The model under review builds one solid part; all positions refer to its coordinate system, in mm. A direction names the side the tool comes from. Round coordinates to 2 decimals unless told otherwise and drop trailing zeros. Loops run counter-clockwise (first coordinate to the right, second up) from the corner with the lowest first, then second, coordinate; pieces in that order, holes last. Notation, with made-up numbers: M 56.25,59 L 92.25,59 A31 ccw 92.25,90 Z; hole C 42.25,-34 d7. An arc over 180 degrees is marked long. Answer as a JSON object with one key per item and string values. Group by question number.
Item 1: The part is to be moulded in two halves that separate along Y. For faces 1 (the face through (83.773, 18.391, 3.285)), 2 (the face through (0.9, 0.86, 18.25)), 3 (the face through (31.1, 51.14, 2.03)), 4 (the face through (85.7, 23.4, 4)), say which applies: +Y half, -Y half, draft (parallel to the pull), parting line (faces both ways), or undercut.
Item 2: To check wall thickness, follow line 1 (Y direction, x = 4, z = 31); line 2 (Y direction, x = 31.5, z = 11); line 3 (X direction, y = 21, z = 15). State the ranges of each line that lie inside material, in increasing order.
Item 3: Consider section A-A (y = 22.5). Give the boundary of the cut face in (x, z), and give its area (3 significant figures).
Item 4: Consider section D-D (y = 42). Give the boundary of the cut face in (x, z).
Item 5: Consider section C-C (x = 38). Give the boundary of the cut face in (y, z).
Item 6: Consider section B-B (z = 26). Give the boundary of the cut face in (x, y), and give its area (3 significant figures).
Item 7: Insertion check: P1, Ø1.2, axis at x = 65, y = 12, coming from the +Z side; P2, Ø0.9, axis at x = 1, z = 30.5, coming from the +Y side; P3, Ø2, axis at x = 65, y = 37, coming from the +Z side. Each pin has a flat end and moves straight along its axis. Give the tip position at first contact, or say it passes through.
Item 8: Tool access review of faces 5 (the face through (26, -5.8, 4)), 6 (the face through (26, 52, 2)), 7 (the face through (20.86, 51.1, 2.03)), 8 (the face through (26, 50.5, 2)), 9 (the face through (77.155, 3.521, 26.14)): name each direction out of +Z, -Z, +X, -X, +Y, -Y from which nothing blocks a thin tool from reaching the whole face with its end or side.
```python
from build123d import *

# Parameters (mm, degrees)
SKETCH_W        = 80
SKETCH_H        = 46
PAD_DEPTH       = 36
SKETCH001_W     = 74
SKETCH001_H     = 40
POCKET_DEPTH    = 33
SKETCH002_W     = 3
SKETCH002_H     = 26.8
POCKET001_DEPTH = 15.9
SKETCH003_R     = 3
PAD001_DEPTH    = 33
SKETCH006_R     = 1.25
POCKET002_DEPTH = 20
SKETCH007_R     = 1.2
PAD002_DEPTH    = 3
SKETCH008_W     = 3.5
SKETCH008_H     = 2
SKETCH008_W_2   = 2
SKETCH008_H_2   = 8
PAD003_DEPTH    = 1
FILLET_R        = 3
FILLET001_R     = 3
FILLET002_R     = 3
SKETCH009_W     = 12
SKETCH009_H     = 6
SKETCH009_W_2   = 6
SKETCH009_H_2   = 12
PAD004_DEPTH    = 4
FILLET003_R     = 1.5
FILLET004_R     = 3
FILLET005_R     = 1.5
FILLET006_R     = 1.5
FILLET007_R     = 1.5
FILLET008_R     = 3
FILLET009_R     = 3
FILLET010_R     = 1.5
FILLET011_R     = 1.5
POCKET003_DEPTH = 4
CHAMFER_SIZE    = 1
CHAMFER001_SIZE = 1
CHAMFER002_SIZE = 1


with BuildPart() as part:
    # Sketch → Pad (new body)
    with BuildSketch(Plane.XY):
        with Locations((40, 23)):
            Rectangle(SKETCH_W, SKETCH_H)
    extrude(amount=PAD_DEPTH)

    # Sketch001 → Pocket (cut)
    with BuildSketch(Plane.XY.offset(36)):
        with Locations((40, 23)):
            Rectangle(SKETCH001_W, SKETCH001_H)
    extrude(amount=-POCKET_DEPTH, mode=Mode.SUBTRACT)

    # Sketch002 → Pocket001 (cut)
    with BuildSketch(Plane.XY.offset(36)):
        with Locations((1.5, 23)):
            Rectangle(SKETCH002_W, SKETCH002_H)
    extrude(amount=-POCKET001_DEPTH, mode=Mode.SUBTRACT)

    # Sketch003 → Pad001 (new body)
    with BuildSketch(Plane.XY.offset(3)):
        with Locations((4, 42)):
            Circle(SKETCH003_R)
        with Locations((4, 4)):
            Circle(SKETCH003_R)
        with Locations((76, 4)):
            Circle(SKETCH003_R)
        with Locations((76, 42)):
            Circle(SKETCH003_R)
    extrude(amount=PAD001_DEPTH)

    # Sketch006 → Pocket002 (cut)
    with BuildSketch(Plane.XY.offset(36)):
        with Locations((4, 42)):
            Circle(SKETCH006_R)
        with Locations((4, 4)):
            Circle(SKETCH006_R)
        with Locations((76, 4)):
            Circle(SKETCH006_R)
        with Locations((76, 42)):
            Circle(SKETCH006_R)
    extrude(amount=-POCKET002_DEPTH, mode=Mode.SUBTRACT)

    # Sketch007 → Pad002 (new body)
    with BuildSketch(Plane.XY.offset(3)):
        with Locations((7, 11.5)):
            Circle(SKETCH007_R)
        with Locations((7, 34.5)):
            Circle(SKETCH007_R)
        with Locations((65, 34.5)):
            Circle(SKETCH007_R)
        with Locations((65, 11.5)):
            Circle(SKETCH007_R)
    extrude(amount=PAD002_DEPTH)

    # Sketch008 → Pad003 (new body)
    with BuildSketch(Plane.XY.offset(3)):
        with Locations((4.75, 34.5)):
            Rectangle(SKETCH008_W, SKETCH008_H)
        with Locations((4.75, 11.5)):
            Rectangle(SKETCH008_W, SKETCH008_H)
        with Locations((65, 39)):
            Rectangle(SKETCH008_W_2, SKETCH008_H_2)
        with Locations((65, 7)):
            Rectangle(SKETCH008_W_2, SKETCH008_H_2)
    extrude(amount=PAD003_DEPTH)

    # Fillet
    fillet_edges = [part.edges().sort_by_distance(p)[0] for p in [
        (80, 0, 18),
    ]]
    fillet(fillet_edges, radius=FILLET_R)

    # Fillet001
    fillet001_edges = [part.edges().sort_by_distance(p)[0] for p in [
        (80, 46, 18),
    ]]
    fillet(fillet001_edges, radius=FILLET001_R)

    # Fillet002
    fillet002_edges = [part.edges().sort_by_distance(p)[0] for p in [
        (0, 0, 18),
        (0, 46, 18),
    ]]
    fillet(fillet002_edges, radius=FILLET002_R)

    # Sketch009 → Pad004 (new body)
    with BuildSketch(Plane(origin=(0, 0, 0), x_dir=(1, 0, 0), z_dir=(0, 0, -1))):
        with Locations((26, 3)):
            Rectangle(SKETCH009_W, SKETCH009_H)
        with Locations((83, -23)):
            Rectangle(SKETCH009_W_2, SKETCH009_H_2)
        with Locations((26, -49)):
            Rectangle(SKETCH009_W, SKETCH009_H)
    extrude(amount=-PAD004_DEPTH)

    # Fillet003
    fillet003_edges = [part.edges().sort_by_distance(p)[0] for p in [
        (26, 46, 4),
        (32, 46, 2),
    ]]
    fillet(fillet003_edges, radius=FILLET003_R)

    # Fillet004
    fillet004_edges = [part.edges().sort_by_distance(p)[0] for p in [
        (32, 52, 2),
        (20, 52, 2),
    ]]
    fillet(fillet004_edges, radius=FILLET004_R)

    # Fillet005
    fillet005_edges = [part.edges().sort_by_distance(p)[0] for p in [
        (20, 46, 2),
    ]]
    fillet(fillet005_edges, radius=FILLET005_R)

    # Fillet006
    fillet006_edges = [part.edges().sort_by_distance(p)[0] for p in [
        (80, 23, 4),
        (80, 29, 2),
    ]]
    fillet(fillet006_edges, radius=FILLET006_R)

    # Fillet007
    fillet007_edges = [part.edges().sort_by_distance(p)[0] for p in [
        (80, 17, 2),
    ]]
    fillet(fillet007_edges, radius=FILLET007_R)

    # Fillet008
    fillet008_edges = [part.edges().sort_by_distance(p)[0] for p in [
        (86, 17, 2),
        (86, 29, 2),
    ]]
    fillet(fillet008_edges, radius=FILLET008_R)

    # Fillet009
    fillet009_edges = [part.edges().sort_by_distance(p)[0] for p in [
        (32, -6, 2),
        (20, -6, 2),
    ]]
    fillet(fillet009_edges, radius=FILLET009_R)

    # Fillet010
    fillet010_edges = [part.edges().sort_by_distance(p)[0] for p in [
        (26, 0, 4),
        (32, 0, 2),
    ]]
    fillet(fillet010_edges, radius=FILLET010_R)

    # Fillet011
    fillet011_edges = [part.edges().sort_by_distance(p)[0] for p in [
        (20, 0, 2),
    ]]
    fillet(fillet011_edges, radius=FILLET011_R)

    # Sketch010 → Pocket003 (cut)
    with BuildSketch(Plane.XY.offset(4)):
        with BuildLine():
            ThreePointArc((23, 50.5), (21.5, 49), (23, 47.5))
            Line((23, 47.5), (29, 47.5))
            ThreePointArc((29, 47.5), (30.5, 49), (29, 50.5))
            Line((23, 50.5), (29, 50.5))
        make_face()
        with BuildLine():
            ThreePointArc((23, -1.5), (21.5, -3), (23, -4.5))
            Line((23, -4.5), (29, -4.5))
            ThreePointArc((29, -4.5), (30.5, -3), (29, -1.5))
            Line((23, -1.5), (29, -1.5))
        make_face()
        with BuildLine():
            ThreePointArc((84.5, 26), (83, 27.5), (81.5, 26))
            Line((81.5, 26), (81.5, 20))
            ThreePointArc((81.5, 20), (83, 18.5), (84.5, 20))
            Line((84.5, 26), (84.5, 20))
        make_face()
    extrude(amount=-POCKET003_DEPTH, mode=Mode.SUBTRACT)

    # Chamfer
    chamfer_edges = [part.edges().sort_by_distance(p)[0] for p in [
        (21.5, 49, 4),
        (29, 47.5, 2),
        (30.5, 49, 4),
        (26, 47.5, 4),
    ]]
    chamfer(chamfer_edges, length=CHAMFER_SIZE)

    # Chamfer001
    chamfer001_edges = [part.edges().sort_by_distance(p)[0] for p in [
        (26, -1.5, 4),
        (26, -4.5, 4),
        (21.5, -3, 4),
        (29, -4.5, 2),
    ]]
    chamfer(chamfer001_edges, length=CHAMFER001_SIZE)

    # Chamfer002
    chamfer002_edges = [part.edges().sort_by_distance(p)[0] for p in [
        (83, 27.5, 4),
        (84.5, 23, 4),
        (81.5, 23, 4),
        (83, 18.5, 4),
    ]]
    chamfer(chamfer002_edges, length=CHAMFER002_SIZE)


solid = part.part
```
Geometry results:
{
 "1": {"face 1": "undercut", "face 2": "-Y half", "face 3": "+Y half", "face 4": "draft"},
 "2": {"line 1": "y = 0 to 2.75, 5.25 to 7, 39 to 40.75, 43.25 to 46", "line 2": "y = 0 to 3, 43 to 46", "line 3": "x = 0 to 3, 77 to 80"},
 "3": {"outline": "M 0,0 L 81.5,0 L 81.5,3 L 80.56,4.33 A1.5 cw 80,5.5 L 80,36 L 77,36 L 77,3 L 3,3 L 3,20.1 L 0,20.1 Z; M 84.5,0 L 86,0 L 86,4 L 85.5,4 L 84.5,3 Z", "area": "402 mm^2"},
 "4": {"outline": "M 0,0 L 80,0 L 80,36 L 77.25,36 L 77.25,16 L 74.75,16 L 74.75,36 L 73,36 L 73,3 L 66,3 L 66,4 L 64,4 L 64,3 L 7,3 L 7,36 L 5.25,36 L 5.25,16 L 2.75,16 L 2.75,36 L 0,36 Z"},
 "5": {"outline": "M 0,0 L 46,0 L 46,36 L 43,36 L 43,3 L 3,3 L 3,36 L 0,36 Z"},
 "6": {"outline": "M 0,3 A3 ccw 3,0 L 77,0 A3 ccw 80,3 L 80,43 A3 ccw 77,46 L 3,46 A3 ccw 0,43 L 0,36.4 L 3,36.4 L 3,39.17 A3 ccw 6.83,43 L 73.17,43 A3 ccw 77,39.17 L 77,6.83 A3 ccw 73.17,3 L 6.83,3 A3 ccw 3,6.83 L 3,9.6 L 0,9.6 Z; hole C 4,4 d2.5; hole C 4,42 d2.5; hole C 76,4 d2.5; hole C 76,42 d2.5", "area": "668 mm^2"},
 "7": {"P1": "stops at z = 6", "P2": "stops at y = 45.57", "P3": "stops at z = 4"},
 "8": {"face 5": "+Z, +X, -X, -Y", "face 6": "+Z, -Z, +X, -X, +Y", "face 7": "+Z, -Z, -X, +Y", "face 8": "+Z, -Z", "face 9": "+Z"}
}
